Geometry: final body of the model. Coordinates: model frame, mm. Round coordinates to 2 decimals unless told otherwise and drop trailing zeros. Loops run counter-clockwise (first coordinate to the right, second up) from the corner with the lowest first, then second, coordinate; pieces in that order, holes last. Notation, with made-up numbers: M -18,46 L 27,46 A19 cw 27,50 Z; hole C -32,31 d3. An arc over 180 degrees is marked long. Return JSON: item names as keys, results as strings.
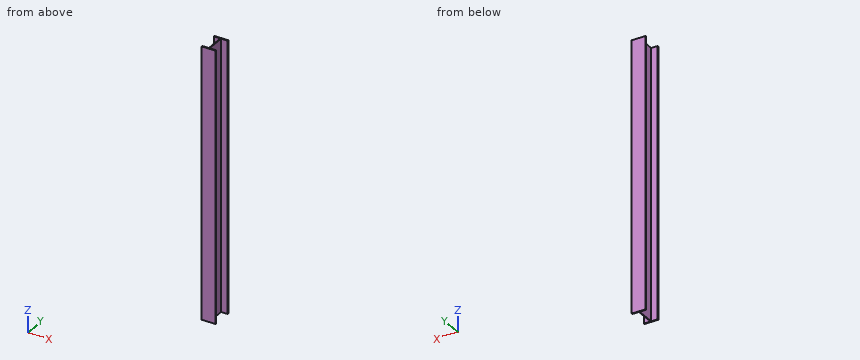
from build123d import *

# Parameters (mm, degrees)
BOSS_EXTRUDE1_DEPTH = 1800
BOSS_EXTRUDE2_DEPTH = 183.1


with BuildPart() as part:
    # Sketch1 → Boss-Extrude1 (new body)
    with BuildSketch(Plane.XY):
        Polygon((0, -0.000240533), (101.6, -0.000240533), (101.6, -7.112240533), (53.408035714, -7.112240533), (53.408035714, -146.050240533), (101.6, -146.050240533), (101.6, -153.162240533), (0, -153.162240533), (0, -146.050240533), (47.566035714, -146.050240533), (47.566035714, -7.112240533), (0, -7.112240533), align=None)
    extrude(amount=BOSS_EXTRUDE1_DEPTH)

    # Sketch3 → Boss-Extrude2 (add)
    with BuildSketch(Plane(origin=(0, 0, 0), x_dir=(-1, 0, 0), z_dir=(0, 0, -1))):
        Polygon((0, -7.112240533), (0, -0.000240533), (-101.6, -0.000240533), (-101.6, -7.112240533), (-53.408035714, -7.112240533), (-53.408035714, -146.050240533), (-101.6, -146.050240533), (-101.6, -153.162240533), (0, -153.162240533), (0, -146.050240533), (-47.566035714, -146.050240533), (-47.566035714, -7.112240533), align=None)
    extrude(amount=BOSS_EXTRUDE2_DEPTH)


solid = part.part
Q1. Section query B-B (z = 1496). Output: boundary loops of the cut face in (x, y).
Determined:
{"outline": "M 0,-153.16 L 101.6,-153.16 L 101.6,-146.05 L 53.41,-146.05 L 53.41,-7.11 L 101.6,-7.11 L 101.6,0 L 0,0 L 0,-7.11 L 47.57,-7.11 L 47.57,-146.05 L 0,-146.05 Z"}
Q2. Material intervals for L1, parallel to Y at x = 84.5, z = 1453; L2, parallel to X at y = -74.5, z = 1365.5, sorted ascending.
Determined:
{"L1": "y = -153.16 to -146.05, -7.11 to 0", "L2": "x = 47.57 to 53.41"}
Q3. Pin query (flat end, axial travel): pin 1 (4 mm diameter, centred on y = -38, z = 1229, fed in from -X). Return the tip coordinate at first contact, or that it passes through.
Determined:
{"pin 1": "stops at x = 47.57"}
Q4. Section query A-A (x = 69). Output: boundary loops of the cut face in (y, z).
Determined:
{"outline": "M -153.16,-183.1 L -146.05,-183.1 L -146.05,1800 L -153.16,1800 Z; M -7.11,-183.1 L 0,-183.1 L 0,1800 L -7.11,1800 Z"}
Q5. Section query C-C (y = -113). Output: boundary loops of the cut face in (x, z).
Determined:
{"outline": "M 47.57,-183.1 L 53.41,-183.1 L 53.41,1800 L 47.57,1800 Z"}
